Autodesk Inventor part; units mm, degrees
ref_plane "YZ Plane" through (0, 0, 0) normal (1, 0, 0) x (0, 1, 0)
ref_plane "XZ Plane" through (0, 0, 0) normal (0, 1, 0) x (-1, 0, 0)
ref_plane "XY Plane" through (0, 0, 0) normal (0, 0, 1) x (1, 0, 0)
sketch "Эскиз1" plane through (0, 0, 0) normal (0, 0, 1) x (1, 0, 0)
  circle A0 centre (0, 0) radius 17.75
  line L0 (0, 0) -> (0, -45)
  circle A1 centre (0, -45) radius 17.75
  line L1 (12.9091, -12.1827) -> (12.9091, -32.8173)
  line L2 (-17.75, 0) -> (-17.75, -45)
  line L3 (9.8694, -14.7532) -> (14.166, -14.7532)
  line L4 (9.8694, -30.2468) -> (17.166, -30.2468)
  line L5 (-16.1446, -7.3766) -> (-17.75, -7.3766)
  line L6 (-16.1446, -37.6234) -> (-17.75, -37.6234)
  line L7 (6.9028, -16.3528) -> (15.2579, -16.3528)
  line L8 (6.9028, -28.6472) -> (17.9028, -28.6472)
  point P0 (12.9091, -30.2468)
  point P1 (12.9091, -14.7532)
  point P2 (12.9091, -28.6472)
  point P3 (12.9091, -16.3528)
  dimension "d0" = 35.5
  dimension "d1" = 45
  dimension "d2" = 35.5
extrude "Выдавливание1" add sketch "Эскиз1" along normal blind 20 contours A0 L0 A1 L6 L2 L5 | A0 L7 L1 L8 A1 L0
properties part number "распорка"
Here's how the part is built. I have some questions about the finished solid (model axes, mm). A direction names the side the tool comes from. Coordinates: 2 decimals unless noted, no trailing zeros. Order: outer loops, then holes, each group sorted by start corner. A loop starts at its lowest first (then second) coordinate and runs counter-clockwise, first axis right, second up.
Item 1: I need wall thicknesses on probe 1 along Y at (x, z) = (8.5, 4); probe 2 along X at (y, z) = (-28.5, 8); probe 3 along X at (y, z) = (-16, 3.5). Which ranges of each line are inside material? Lowest first, please.
Response values:
probe 1: y = -28.65 to -16.35
probe 2: x = -17.75 to -6.54, 6.54 to 12.91
probe 3: x = -17.75 to -7.69
Item 2: I'm going to push flat-ended pins straight in: pin 1 Ø1.5 at (x, z) = (-6, 7.5) entering from -Y; pin 2 Ø1.5 at (x, z) = (8.5, 3) entering from +Y; pin 3 Ø10 at (x, z) = (0.5, 6) entering from +Y. Where does each tip first touch, or does it pass through?
Response values:
pin 1: stops at y = -28.58
pin 2: stops at y = -16.35
pin 3: stops at y = -16.88
Item 3: If we section it at B-B, the plane x = 8.5: List the corners of the cut face in (y, z) for me.
Response values:
outline: (-28.65, 0) - (-16.35, 0) - (-16.35, 20) - (-28.65, 20) - close
Item 4: If we section it at C-C, the plane y = -13: List the corners of the cut face in (x, z) for me.
Response values:
outline: (-17.75, 0) - (-12.09, 0) - (-12.09, 20) - (-17.75, 20) - close
Item 5: If we section it at A-A, the plane z = 8: List the corners of the cut face in (x, y) for me, then the cut area to 3 significant figures.
Response values:
outline: (-17.75, -37.62) - (-16.14, -37.62) arc R17.75 cw to (6.9, -28.65) - (12.91, -28.65) - (12.91, -16.35) - (6.9, -16.35) arc R17.75 cw to (-16.14, -7.38) - (-17.75, -7.38) - close
area: 442 mm2
Item 6: Which directions (+Z, -Z, +X, -X, +Y, -Y) give clear straight access to the entire face, cutting with the end or side of a thin tool? Please do faces 4 (the face through (10, -28.647, 10)), 5 (the face through (-6.26, -16.61, 9.86)), 6 (the face through (10, -16.353, 10)).
Response values:
face 4: +Z, -Z, +X, -Y
face 5: +Z, -Z, +Y
face 6: +Z, -Z, +X, +Y
Item 7: Thinking about a two-plate mould opening in X: for faces 1 (the face through (-6.62, -28.53, 9.86)), 2 (the face through (12.909, -22, 10)), 3 (the face through (-17, -7.377, 10)), which applies, pulls with the +X half, pulls with the -X half, needs draft (parallel to the pull), parting line crosses it, or undercut?
Response values:
face 1: undercut
face 2: pulls with the +X half
face 3: needs draft
